Work out the finished part from the listing and answer in its coordinate system (mm). Face numbers are marked on the shaded views. A direction names the side the tool comes from. Round coordinates to 2 decimals unless told otherwise and drop trailing zeros. Loops run counter-clockwise (first coordinate to the right, second up) from the corner with the lowest first, then second, coordinate; pieces in that order, holes last. Notation, with made-up numbers: (32, 84.25) -> (47, 84.25) arc R10 cw to (47, 90.25) -> close; hole circle Ø7 at (-26, -22). An arc over 180 degrees is marked (long way). Write item = value, one per line. Start each with the question number.
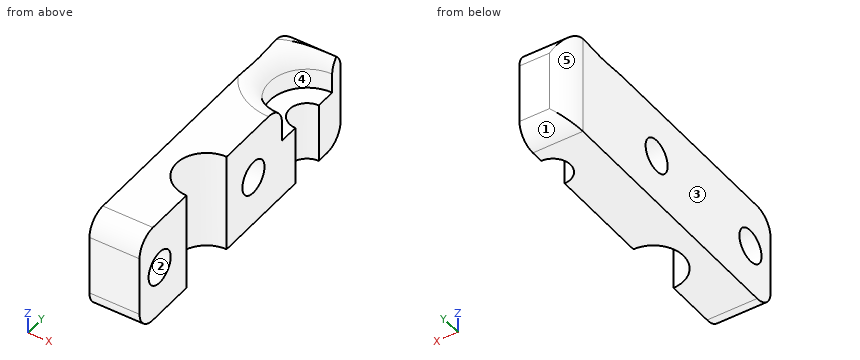
```python
from build123d import *

# Parameters (mm, degrees)
SKETCH_1_W          = 10
SKETCH_1_H          = 20
SKETCH_1_R          = 3
EXTRUDE_1_DEPTH     = 10
SKETCH_2_R          = 1.65
CUT_EXTRUDE_1_DEPTH = 18.320508076
SKETCH_3_W          = 12.852703923
SKETCH_3_H          = 20.2795508
CUT_EXTRUDE_2_DEPTH = 16
EXTRUDE_2_DEPTH     = 10
FILLET_1_R          = 2
SKETCH_6_R          = 3.75
CUT_EXTRUDE_3_DEPTH = 4
FILLET_2_R          = 2


with BuildPart() as part:
    # 草圖1 → 填料-伸長1 (new body)
    with BuildSketch(Plane.XY):
        Rectangle(SKETCH_1_W, SKETCH_1_H)
        Circle(SKETCH_1_R, mode=Mode.SUBTRACT)
    extrude(amount=EXTRUDE_1_DEPTH)

    # 草圖2 → 除料-伸長1 (cut, through all)
    with BuildSketch(Plane.ZY.offset(5)):
        with Locations((5, 7)):
            Circle(SKETCH_2_R)
        with Locations((5, -7)):
            Circle(SKETCH_2_R)
    extrude(amount=-CUT_EXTRUDE_1_DEPTH, mode=Mode.SUBTRACT)

    # 草圖3 → 除料-伸長2 (cut, through all)
    with BuildSketch(Plane.XY.offset(10)):
        with Locations((6.426351961, -0.1397754)):
            Rectangle(SKETCH_3_W, SKETCH_3_H)
    extrude(amount=-CUT_EXTRUDE_2_DEPTH, mode=Mode.SUBTRACT)

    # 草圖5 → 填料-伸長2 (add, through all)
    with BuildSketch(Plane.XY.offset(10)):
        with BuildLine():
            Line((0, 10), (0, 13.25))
            ThreePointArc((0, 13.25), (-1.75, 15), (0, 16.75))
            Line((0, 16.75), (0, 20))
            Line((0, 20), (-5, 20))
            Line((-5, 20), (-5, 10))
            Line((-5, 10), (0, 10))
        make_face()
    extrude(amount=-EXTRUDE_2_DEPTH)

    # 圓角1
    fillet_1_edges = [part.edges().sort_by_distance(p)[0] for p in [
        (-2.5, -10, 0),
        (-2.5, 20, 0),
        (-5, 20, 5),
        (-2.5, 20, 10),
        (-2.5, -10, 10),
    ]]
    fillet(fillet_1_edges, radius=FILLET_1_R)

    # 草圖6 → 除料-伸長3 (cut)
    with BuildSketch(Plane.XY.offset(10)):
        with Locations((0, 15)):
            Circle(SKETCH_6_R)
    extrude(amount=-CUT_EXTRUDE_3_DEPTH, mode=Mode.SUBTRACT)

    # 圓角2
    # the kernel refuses this fillet: 2 mm, written as the material it takes off along each edge
    with BuildSketch(Plane(origin=(0, 15, 10), x_dir=(0.6374525530296073, 0.7704896122830182, 0), z_dir=(0.7704896122830182, -0.6374525530296073, 0))) as fillet_2_piece_1:
        with BuildLine():
            CenterArc((3.75 + FILLET_2_R, -FILLET_2_R), FILLET_2_R, 90, 90)
            Line((3.75, -FILLET_2_R), (3.75, 0))
            Line((3.75, 0), (3.75 + FILLET_2_R, 0))
        make_face()
    revolve(axis=Axis((0, 15, 10), (0, 0, 1)), revolution_arc=296.074145673, mode=Mode.SUBTRACT)


solid = part.part
```
Item 1: The mould has two halves that part along Y. Classify the marked faces 1, 2 and 3: pulls with the +Y half, pulls with the -Y half, needs draft (parallel to the pull), parting line crosses it, or undercut.
Item 2: Flat-ended cylindrical pins translate along their axes: pin 1 (4 mm diameter, centred on y = -7, z = 5, fed in from +X); pin 2 (1.1 mm diameter, centred on x = -2, y = 16, fed in from +Z); pin 3 (3 mm diameter, centred on x = -2, y = 12.5, fed in from +Z). Find the tip coordinate at first contact, or state that the pin passes through.
Item 3: Find the intervals of material crossed by line 1 along Y through (x, z) = (-3.1, 5); line 2 along Y through (x, z) = (-3.9, 5); line 3 along Y through (x, z) = (-1.3, 4), in increasing order. Write a range as [from, to].
Item 4: Section D-D (z = 7.25) is taken. Determine the outline of the cut face in (x, y).
Item 5: Section B-B (y = 7) is taken. Determine the outline of the cut face in (x, z).
Item 6: Section C-C (x = -1.4) is taken. Count the separate pieces of the cut face and the enclosed holes in it, then the cut area to 3 significant figures.
Item 7: A tool of negligible diameter and unlimited length cuts with its end or side. For the marked faces 4 and 5, from which of +Z, -Z, +X, -X, +Y, -Y can it reach the whole face along a straight path? Write none if from no direction.
Item 8: Section A-A (z = 5) is taken. Determine the outline of the cut face in (x, y).
Worked answers:
q1.face_1 = pulls with the +Y half
q1.face_2 = undercut
q1.face_3 = needs draft
q2.pin_1 = 0
q2.pin_2 = 6
q2.pin_3 = 9.7
q3.line_1 = [-10, -8.65], [-5.35, 5.35], [8.65, 20]
q3.line_2 = [-10, -8.65], [-5.35, 5.35], [8.65, 19.79]
q3.line_3 = [-10, -8.31], [-5.69, -2.7], [2.7, 5.69], [8.31, 13.83], [16.17, 20]
q4.outline = (-5, -10) -> (0, -10) -> (0, -3) arc R3 cw to (0, 3) -> (0, 11.25) arc R3.75 cw to (0, 18.75) -> (0, 20) -> (-3, 20) arc R2 ccw to (-5, 18) -> close
q5.outline = (-5, 0) -> (0, 0) -> (0, 3.35) -> (-5, 3.35) -> close; (-5, 6.65) -> (0, 6.65) -> (0, 10) -> (-5, 10) -> close
q6.separate_pieces = 3
q6.enclosed_holes = 2
q6.area = 185 mm2
q7.face_4 = +Z, +X
q7.face_5 = +Z, -Z, -X, +Y
q8.outline = (-5, -10) -> (0, -10) -> (0, -8.65) -> (-5, -8.65) -> close; (-5, -5.35) -> (0, -5.35) -> (0, -3) arc R3 cw to (0, 3) -> (0, 5.35) -> (-5, 5.35) -> close; (-5, 8.65) -> (0, 8.65) -> (0, 13.25) arc R1.75 cw to (0, 16.75) -> (0, 20) -> (-3, 20) arc R2 ccw to (-5, 18) -> close
